For this review, take the finished solid that the model builds, in its own axes (mm). A direction names the side the tool comes from. Coordinates: 2 decimals unless noted, no trailing zeros. Order: outer loops, then holes, each group sorted by start corner. A loop starts at its lowest first (then second) coordinate and runs counter-clockwise, first axis right, second up.
from build123d import *

# Parameters (mm, degrees)
SKETCH_1_W      = 33.7
SKETCH_1_H      = 26.7
SKETCH_1_R      = 1.500160794
SKETCH_1_R_2    = 1.5
SKETCH_1_R_3    = 1.552324123
SKETCH_1_R_4    = 1.546482565
EXTRUDE_1_DEPTH = 1.3
SKETCH_2_W      = 2.597810981
SKETCH_2_H      = 12.596422695
EXTRUDE_3_DEPTH = 2.6
SKETCH_3_W      = 0.801502227
SKETCH_3_H      = 0.800416217
SKETCH_3_H_2    = 0.802091773
SKETCH_3_H_3    = 0.798469443
SKETCH_3_H_4    = 0.802947908
SKETCH_3_H_5    = 0.804334784
SKETCH_6_W      = 16.101670469
SKETCH_6_H      = 16.19878198
EXTRUDE_4_DEPTH = 12.4
SKETCH_7_R      = 13.101940721
EXTRUDE_5_DEPTH = 8.4
FILLET_1_R      = 7.85
SKETCH_9_R      = 5.251940721
EXTRUDE_6_DEPTH = 5.3
SKETCH_12_R     = 9.651169133
EXTRUDE_8_DEPTH = 4.6
FILLET_2_R      = 3.5


with BuildPart() as part:
    # Эскиз1 → Бобышка-Вытянуть1 (new body)
    with BuildSketch(Plane(origin=(0, 0, 0), x_dir=(1, 0, 0), z_dir=(0, 1, 0))):
        with Locations((16.85, 13.35)):
            Rectangle(SKETCH_1_W, SKETCH_1_H)
        with Locations(Location((30.998263896, 3.498646338, 0), (0, 0, 270))):
            Circle(SKETCH_1_R, mode=Mode.SUBTRACT)
        with Locations(Location((30.998263896, 23.098469173, 0), (0, 0, 270))):
            Circle(SKETCH_1_R_2, mode=Mode.SUBTRACT)
        with Locations(Location((5.150482455, 3.352746683, 0), (0, 0, 270))):
            Circle(SKETCH_1_R_3, mode=Mode.SUBTRACT)
        with Locations(Location((5.150482455, 22.950000581, 0), (0, 0, 270))):
            Circle(SKETCH_1_R_4, mode=Mode.SUBTRACT)
    extrude(amount=EXTRUDE_1_DEPTH)

    # Эскиз2 → Бобышка-Вытянуть3 (add)
    with BuildSketch(Plane.XZ):
        with Locations((2.697533257, -12.993800664)):
            Rectangle(SKETCH_2_W, SKETCH_2_H)
    extrude(amount=EXTRUDE_3_DEPTH)

    # По траектории3: sweep along a path in Эскиз4
    with BuildLine(Plane.XY) as sweep_3_path:
        Line((2.697117024, -2.6), (2.697117024, -3.4))
        ThreePointArc((2.697117024, -3.4), (2.404223805, -4.107106781), (1.697117024, -4.4))
        Line((1.697117024, -4.4), (-4.903035907, -4.4))
    # Эскиз3 → По траектории3 (sweep)
    with BuildSketch(Plane.XZ.offset(2.6)):
        with Locations((2.697117024, -18.090816879)):
            Rectangle(SKETCH_3_W, SKETCH_3_H)
        with Locations((2.697117024, -15.69317288)):
            Rectangle(SKETCH_3_W, SKETCH_3_H_2)
        with Locations((2.697117024, -13.090941171)):
            Rectangle(SKETCH_3_W, SKETCH_3_H_3)
        with Locations((2.697117024, -10.688983068)):
            Rectangle(SKETCH_3_W, SKETCH_3_H_4)
        with Locations((2.697117024, -8.082021693)):
            Rectangle(SKETCH_3_W, SKETCH_3_H_5)
    sweep(path=sweep_3_path.line)

    # Эскиз6 → Бобышка-Вытянуть4 (add)
    with BuildSketch(Plane.XZ):
        with Locations((17.251381143, -12.805593049)):
            Rectangle(SKETCH_6_W, SKETCH_6_H)
    extrude(amount=EXTRUDE_4_DEPTH)

    # Эскиз7 → Бобышка-Вытянуть5 (add)
    with BuildSketch(Plane.XZ.offset(12.4)):
        with Locations(Location((17.251381142, -12.805593049, 0), (0, 0, 270))):
            Circle(SKETCH_7_R)
    extrude(amount=EXTRUDE_5_DEPTH)

    # Скругление1
    fillet_1_edges = [part.edges().sort_by_distance(p)[0] for p in [
        (17.251381142, -20.8, 0.296347672),
    ]]
    fillet(fillet_1_edges, radius=FILLET_1_R)

    # Эскиз9 → Бобышка-Вытянуть6 (add)
    with BuildSketch(Plane.XZ.offset(20.8)):
        with Locations(Location((17.251381142, -12.805593049, 0), (0, 0, 270))):
            Circle(SKETCH_9_R)
    extrude(amount=EXTRUDE_6_DEPTH)

    # Эскиз12 → Бобышка-Вытянуть8 (add)
    with BuildSketch(Plane.XZ.offset(26.1)):
        with Locations(Location((17.236348133, -12.810976669, 0), (0, 0, 270))):
            Circle(SKETCH_12_R)
    extrude(amount=EXTRUDE_8_DEPTH)

    # Скругление2
    fillet_2_edges = [part.edges().sort_by_distance(p)[0] for p in [
        (17.236348133, -30.7, -3.159807536),
    ]]
    fillet(fillet_2_edges, radius=FILLET_2_R)


solid = part.part
1. Machinability: for faces 1 (the face through (13, -26.1, -17)), 2 (the face through (3, -1, -19.292)), 3 (the face through (-0.1, -4.2, -13.49)), 4 (the face through (2.7, -4.38, -18.09)), 5 (the face through (1.399, -1, -13)), which of the approach directions +Z, -Z, +X, -X, +Y, -Y give a long, thin tool a straight path to every point of the face, cutting with its end or side? Answer none if there is none.
Answer below:
face 1: none
face 2: -Z, -X, -Y
face 3: -X, -Y
face 4: +Z, -Z, -Y
face 5: +Z, -Z, -X
2. The part is to be moulded in two halves that separate along Y. For faces 6 (the face through (17, -6, -20.905)), 7 (the face through (2.7, -4.38, -8.08)), 8 (the face through (5.628, -12.671, -18.851)), say which applies: +Y half, -Y half, draft (parallel to the pull), parting line (faces both ways), or undercut.
Answer below:
face 6: undercut
face 7: -Y half
face 8: draft
3. Take a section at B-B, the plane z = -23. Give the number of separate pieces and of enclosed holes in the cut face, plus the area to 3 significant figures.
Answer below:
separate pieces: 4
enclosed holes: 0
area: 125 mm2
4. Take a section at A-A, the plane y = -11.5. Give the boundary of the cut face in (x, z), plus the area to 3 significant figures.
Answer below:
outline: (9.2, -20.9) - (25.3, -20.9) - (25.3, -4.71) - (9.2, -4.71) - close
area: 261 mm2
5. Clearance check with flat-ended pins moving along their axes: pin 1 Ø6 at (y, z) = (-18, -24) entering from -X; pin 2 Ø10 at (x, y) = (1.5, -6) entering from +Z; pin 3 Ø4 at (x, z) = (31, -23.1) entering from -Y. State where each tip first meets the part, or that it passes through.
Answer below:
pin 1: stops at x = 8.51
pin 2: stops at z = -6.7
pin 3: stops at y = 0
6. To check wall thickness, follow L1, parallel to X at y = 0.5, z = -22.95; L2, parallel to Y at x = 1, z = -8.25; L3, parallel to Y at x = 13, z = -9.5. State the ranges of each line that lie inside material, in increasing order.
Answer below:
L1: x = 0 to 3.6, 6.7 to 29.51, 32.49 to 33.7
L2: y = -4.8 to -4, 0 to 1.3
L3: y = -30.7 to -26.1, -20.8 to 1.3
